Can you work these out from the model? Positions are in its coordinate system, mm. A direction names the side the tool comes from. Give positions to 0.01 mm unless a question says otherwise; leave off trailing zeros. Write each loop counter-clockwise with the first axis right and the second up, starting at its lowest first coordinate (ties: lowest second). Pieces come first, ordered by that corner, then holes. Notation, with made-up numbers: M 58,48.5 L 65,48.5 A20 cw 65,82.5 Z; hole C 11,24.5 d8. An arc over 180 degrees is marked long. Write each question's results on one line, items separated by ' | '.
from build123d import *

# Parameters (mm, degrees)
F1_DEPTH = 12.7


with BuildPart() as f1:
    # F0 (on Front) → F1 (new body)
    with BuildSketch(Plane.XZ):
        with BuildLine():
            ThreePointArc((3.5606706706, -0.7425834457), (3.6180769765, -0.3732623619), (3.63728, 0))
            ThreePointArc((3.63728, 0), (3.6213765163, 0.3397615722), (3.5738051364, 0.6765520271))
            ThreePointArc((3.5738051364, 0.6765520271), (3.4825423587, 1.0496211309), (3.3524499928, 1.4109871879))
            ThreePointArc((3.3524499928, 1.4109871879), (3.2108553593, 1.7088632654), (3.0428601668, 1.9926885867))
            ThreePointArc((3.0428601668, 1.9926885867), (2.7896517807, 2.3340198673), (2.498357335, 2.6434856582))
            ThreePointArc((2.498357335, 2.6434856582), (2.2807047164, 2.8334063942), (2.0486673204, 3.0054563728))
            ThreePointArc((2.0486673204, 3.0054563728), (1.7124143827, 3.2089628823), (1.3561660359, 3.3749991824))
            ThreePointArc((1.3561660359, 3.3749991824), (1.0534732185, 3.4813790337), (0.7425834457, 3.5606706706))
            Line((0.7425834457, 3.5606706706), (0, 3.63728))
            ThreePointArc((0, 3.63728), (-0.3397615722, 3.6213765163), (-0.6765520271, 3.5738051364))
            ThreePointArc((-0.6765520271, 3.5738051364), (-0.7247312416, 3.5643471248), (-0.7727783981, 3.5542396298))
            ThreePointArc((-0.7727783981, 3.5542396298), (-1.0444322734, 3.4841020399), (-1.3098719531, 3.3932346316))
            ThreePointArc((-1.3098719531, 3.3932346316), (-1.6605472279, 3.2361070289), (-1.9926885867, 3.0428601668))
            ThreePointArc((-1.9926885867, 3.0428601668), (-2.2476575865, 2.8596924961), (-2.4858819563, 2.6552206496))
            ThreePointArc((-2.4858819563, 2.6552206496), (-2.7623678061, 2.3662480643), (-3.0054563728, 2.0486673204))
            ThreePointArc((-3.0054563728, 2.0486673204), (-3.1608520437, 1.7996722357), (-3.2956657104, 1.5389585191))
            ThreePointArc((-3.2956657104, 1.5389585191), (-3.451215794, 1.1484403953), (-3.5606706706, 0.7425834457))
            ThreePointArc((-3.5606706706, 0.7425834457), (-3.6180769765, 0.3732623619), (-3.63728, 0))
            ThreePointArc((-3.63728, 0), (-3.6213765163, -0.3397615722), (-3.5738051364, -0.6765520271))
            ThreePointArc((-3.5738051364, -0.6765520271), (-3.4978828331, -0.9973071162), (-3.3932346316, -1.3098719531))
            ThreePointArc((-3.3932346316, -1.3098719531), (-3.2361070289, -1.6605472279), (-3.0428601668, -1.9926885867))
            ThreePointArc((-3.0428601668, -1.9926885867), (-2.8015066019, -2.3197772647), (-2.5251625854, -2.6178922277))
            ThreePointArc((-2.5251625854, -2.6178922277), (-2.2951103445, -2.8217502202), (-2.0486673204, -3.0054563728))
            ThreePointArc((-2.0486673204, -3.0054563728), (-1.7010031558, -3.2150262927), (-1.332151365, -3.3845499759))
            ThreePointArc((-1.332151365, -3.3845499759), (-1.0410983424, -3.4850997174), (-0.7425834457, -3.5606706706))
            ThreePointArc((-0.7425834457, -3.5606706706), (-0.3732623619, -3.6180769765), (0, -3.63728))
            ThreePointArc((0, -3.63728), (0.3397615722, -3.6213765163), (0.6765520271, -3.5738051364))
            ThreePointArc((0.6765520271, -3.5738051364), (1.1064219136, -3.4649150563), (1.5198461677, -3.3045231767))
            ThreePointArc((1.5198461677, -3.3045231767), (1.7611337209, -3.1824854777), (1.9926885867, -3.0428601668))
            ThreePointArc((1.9926885867, -3.0428601668), (2.4072483422, -2.7267125293), (2.7723506783, -2.3545440142))
            ThreePointArc((2.7723506783, -2.3545440142), (2.8929489657, -2.2046886584), (3.0054563728, -2.0486673204))
            ThreePointArc((3.0054563728, -2.0486673204), (3.2607503405, -1.6116181357), (3.4529018963, -1.1433609635))
            ThreePointArc((3.4529018963, -1.1433609635), (3.5125070381, -0.9445105112), (3.5606706706, -0.7425834457))
        make_face()
        with BuildLine():
            Line((4.6645724086, -0.514333969), (3.63728, 0))
            ThreePointArc((3.63728, 0), (3.6180769765, -0.3732623619), (3.5606706706, -0.7425834457))
            Line((3.5606706706, -0.7425834457), (4.6645724086, -0.514333969))
        make_face()
        with BuildLine():
            ThreePointArc((3.3524499928, 1.4109871879), (3.4825423587, 1.0496211309), (3.5738051364, 0.6765520271))
            Line((3.5738051364, 0.6765520271), (4.5063300649, 1.3098719531))
            Line((4.5063300649, 1.3098719531), (3.3524499928, 1.4109871879))
        make_face()
        with BuildLine():
            Line((4.1126758876, -2.2602372067), (3.4529018963, -1.1433609635))
            ThreePointArc((3.4529018963, -1.1433609635), (3.2607503405, -1.6116181357), (3.0054563728, -2.0486673204))
            Line((3.0054563728, -2.0486673204), (4.1126758876, -2.2602372067))
        make_face()
        with BuildLine():
            ThreePointArc((2.498357335, 2.6434856582), (2.7896517807, 2.3340198673), (3.0428601668, 1.9926885867))
            Line((3.0428601668, 1.9926885867), (3.6620398187, 2.9346617442))
            Line((3.6620398187, 2.9346617442), (2.498357335, 2.6434856582))
        make_face()
        with BuildLine():
            Line((2.9346617442, -3.6620398187), (2.7723506783, -2.3545440142))
            ThreePointArc((2.7723506783, -2.3545440142), (2.4072483422, -2.7267125293), (1.9926885867, -3.0428601668))
            Line((1.9926885867, -3.0428601668), (2.9346617442, -3.6620398187))
        make_face()
        with BuildLine():
            ThreePointArc((1.3561660359, 3.3749991824), (1.7124143827, 3.2089628823), (2.0486673204, 3.0054563728))
            Line((2.0486673204, 3.0054563728), (2.2602372067, 4.1126758876))
            Line((2.2602372067, 4.1126758876), (1.3561660359, 3.3749991824))
        make_face()
        with BuildLine():
            Line((1.3098719531, -4.5063300649), (1.5198461677, -3.3045231767))
            ThreePointArc((1.5198461677, -3.3045231767), (1.1064219136, -3.4649150563), (0.6765520271, -3.5738051364))
            Line((0.6765520271, -3.5738051364), (1.3098719531, -4.5063300649))
        make_face()
        with BuildLine():
            Line((0, 3.63728), (0.7425834457, 3.5606706706))
            ThreePointArc((0.7425834457, 3.5606706706), (0.3732623619, 3.6180769765), (0, 3.63728))
        make_face()
        with BuildLine():
            ThreePointArc((0, 3.63728), (0.3732623619, 3.6180769765), (0.7425834457, 3.5606706706))
            Line((0.7425834457, 3.5606706706), (0.514333969, 4.6645724086))
            Line((0.514333969, 4.6645724086), (0, 3.63728))
        make_face()
        with BuildLine():
            Line((-0.514333969, -4.6645724086), (0, -3.63728))
            ThreePointArc((0, -3.63728), (-0.3732623619, -3.6180769765), (-0.7425834457, -3.5606706706))
            Line((-0.7425834457, -3.5606706706), (-0.514333969, -4.6645724086))
        make_face()
        with BuildLine():
            ThreePointArc((-0.7727783981, 3.5542396298), (-0.7247312416, 3.5643471248), (-0.6765520271, 3.5738051364))
            Line((-0.6765520271, 3.5738051364), (-1.3098719531, 4.5063300649))
            Line((-1.3098719531, 4.5063300649), (-1.3098719531, 3.8332852884))
            Line((-1.3098719531, 3.8332852884), (-0.7727783981, 3.5542396298))
        make_face()
        with BuildLine():
            ThreePointArc((-1.3098719531, 3.3932346316), (-1.0444322734, 3.4841020399), (-0.7727783981, 3.5542396298))
            Line((-0.7727783981, 3.5542396298), (-1.3098719531, 3.8332852884))
            Line((-1.3098719531, 3.8332852884), (-1.3098719531, 3.3932346316))
        make_face()
        with BuildLine():
            Line((-2.2602372067, -4.1126758876), (-1.332151365, -3.3845499759))
            ThreePointArc((-1.332151365, -3.3845499759), (-1.7010031558, -3.2150262927), (-2.0486673204, -3.0054563728))
            Line((-2.0486673204, -3.0054563728), (-2.2602372067, -4.1126758876))
        make_face()
        with BuildLine():
            ThreePointArc((-2.4858819563, 2.6552206496), (-2.2476575865, 2.8596924961), (-1.9926885867, 3.0428601668))
            Line((-1.9926885867, 3.0428601668), (-2.9346617442, 3.6620398187))
            Line((-2.9346617442, 3.6620398187), (-2.4858819563, 2.6552206496))
        make_face()
        with BuildLine():
            Line((-3.6620398187, -2.9346617442), (-2.5251625854, -2.6178922277))
            ThreePointArc((-2.5251625854, -2.6178922277), (-2.8015066019, -2.3197772647), (-3.0428601668, -1.9926885867))
            Line((-3.0428601668, -1.9926885867), (-3.6620398187, -2.9346617442))
        make_face()
        with BuildLine():
            ThreePointArc((-3.2956657104, 1.5389585191), (-3.1608520437, 1.7996722357), (-3.0054563728, 2.0486673204))
            Line((-3.0054563728, 2.0486673204), (-4.1126758876, 2.2602372067))
            Line((-4.1126758876, 2.2602372067), (-3.2956657104, 1.5389585191))
        make_face()
        with BuildLine():
            Line((-4.5063300649, -1.3098719531), (-3.3932346316, -1.3098719531))
            ThreePointArc((-3.3932346316, -1.3098719531), (-3.4978828331, -0.9973071162), (-3.5738051364, -0.6765520271))
            Line((-3.5738051364, -0.6765520271), (-4.5063300649, -1.3098719531))
        make_face()
        with BuildLine():
            ThreePointArc((-3.63728, 0), (-3.6180769765, 0.3732623619), (-3.5606706706, 0.7425834457))
            Line((-3.5606706706, 0.7425834457), (-4.6645724086, 0.514333969))
            Line((-4.6645724086, 0.514333969), (-3.63728, 0))
        make_face()
    extrude(amount=F1_DEPTH)


solid = f1.part
Item 1: I'm going to push flat-ended pins straight in: pin 1 (1.5 mm diameter, centred on y = -9.5, z = -1.5, fed in from -X); pin 2 (1.2 mm diameter, centred on x = -4, y = -7.5, fed in from -Z); pin 3 (0.6 mm diameter, centred on y = -9.5, z = 4, fed in from -X). Where does each tip first touch, or does it pass through?
Geometry says:
pin 1: stops at x = -4.51 | pin 2: stops at z = -2.93 | pin 3: stops at x = -1.31
Item 2: For faces 5 (the face through (-0.989, -6.261, 4.034)), 6 (the face through (-4.1, -6.26, 0.63)), 7 (the face through (-1.8, -6.26, -3.75)), 8 (the face through (4.1, -6.26, -0.63)), which set-ups out of +Z, -Z, +X, -X, +Y, -Y let a thin tool reach every point of the face, with its end or its side?
Geometry says:
face 5: +Z, +Y, -Y | face 6: -X, +Y, -Y | face 7: -Z, +Y, -Y | face 8: +X, +Y, -Y
Item 3: Thinking about a two-plate mould opening in Z: for faces 1 (the face through (-4.16, -6.26, 0.26)), 2 (the face through (2.153, -6.261, 3.551)), 3 (the face through (0, -12.7, 0)), 4 (the face through (-0.26, -6.26, -4.16)), which applies, +Z half, -Z half, draft (parallel to the pull), parting line (faces both ways), or undercut?
Geometry says:
face 1: undercut | face 2: undercut | face 3: draft | face 4: -Z half
Item 4: I want a section at B-B, the plane x = -1.75. Please give me the cut outline in (y, z), and give its area (3 significant figures).
Geometry says:
outline: M -12.7,-3.71 L 0,-3.71 L 0,3.19 L -12.7,3.19 Z | area: 87.6 mm2
Item 5: If I drill on line 1 (Z direction, x = 3.75, y = -5.75); line 2 (Z direction, x = 4, y = -1.5); line 3 (Z direction, x = -3.25, y = -5.25), over which ranges is the centre line in solid material (lowest first)? Write a range as from..to.
Geometry says:
line 1: z = -2.19..-1.65, -0.7..-0.06, 0.8..1.38 | line 2: z = -2.24..-2.07, -0.65..-0.18, 0.97..1.35 | line 3: z = -2.82..-2.31, -1.63..2.1
Item 6: I want a section at A-A, the plane x = -0.25. Please give me the cut outline in (y, z), and give its area (3 significant figures).
Geometry says:
outline: M -12.7,-4.14 L 0,-4.14 L 0,3.63 L -12.7,3.63 Z | area: 98.6 mm2
